```python
from build123d import *

# Parameters (mm, degrees)
F0_W     = 74
F0_H     = 32
F1_DEPTH = 3.4
F2_W     = 68.8
F2_H     = 27.8
F3_DEPTH = 10
F4_W     = 65.06
F4_H     = 24.6
F5_DEPTH = 8
F6_R     = 5
F7_R     = 1.6
F8_DEPTH = 10.001
F9_R     = 1


with BuildPart() as f1:
    # F0 (on Top) → F1 (new body)
    with BuildSketch(Plane.XY):
        Rectangle(F0_W, F0_H)
    extrude(amount=F1_DEPTH)

    # F2 (on face) → F3 (join)
    with BuildSketch(Plane.XY.offset(3.4)):
        Rectangle(F2_W, F2_H)
    extrude(amount=-F3_DEPTH)

    # F4 (on face) → F5 (cut)
    with BuildSketch(Plane.XY.offset(3.4)):
        Rectangle(F4_W, F4_H)
    extrude(amount=-F5_DEPTH, mode=Mode.SUBTRACT)

    # F6
    f6_edges = [f1.edges().sort_by_distance(p)[0] for p in [
        (-37, -16, 1.7),
        (37, -16, 1.7),
        (37, 16, 1.7),
        (-37, 16, 1.7),
    ]]
    fillet(f6_edges, radius=F6_R)

    # F7 (on face) → F8 (cut, through all)
    with BuildSketch(Plane.XY.offset(3.4)):
        with Locations((-30.004807, -10.013314)):
            Circle(F7_R)
    extrude(amount=-F8_DEPTH, mode=Mode.SUBTRACT)

    # F9
    f9_edges = [f1.edges().sort_by_distance(p)[0] for p in [
        (-34.4, 13.9, -3.3),
        (-34.4, -13.9, -3.3),
        (34.4, -13.9, -3.3),
        (34.4, 13.9, -3.3),
    ]]
    fillet(f9_edges, radius=F9_R)


solid = f1.part
```
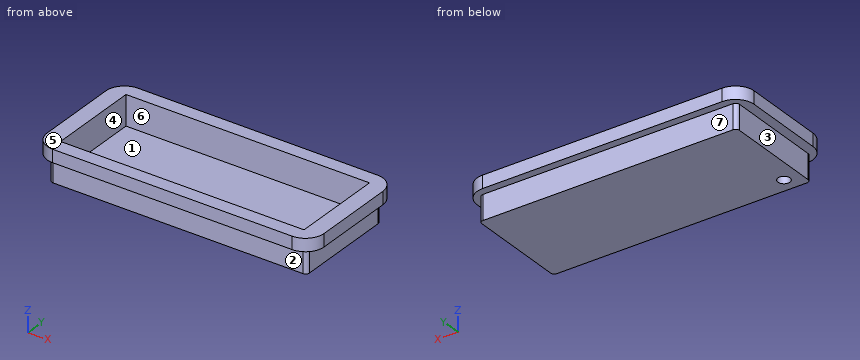
The model under review builds one solid part; all positions refer to its coordinate system, in mm. Face numbers are marked on the shaded views. A direction names the side the tool comes from. Round coordinates to 2 decimals unless told otherwise and drop trailing zeros. Write each loop counter-clockwise with the first axis right and the second up, starting at its lowest first coordinate (ties: lowest second). Pieces come first, ordered by that corner, then holes. Notation, with made-up numbers: (-26.5, 19.25) -> (15.5, 19.25) arc R13 cw to (15.5, 37.25) -> close; hole circle Ø8 at (69, 9.25). An arc over 180 degrees is marked (long way). Use CSV: the item, a comma, the result in double quotes.
Q1. To check wall thickness, follow probe 1 along X at (y, z) = (-2, -3); probe 2 along Y at (x, z) = (-14.5, -1.5); probe 3 along X at (y, z) = (0, 1.75). State the ranges of each line that lie inside material, in increasing order. Write a range as [from, to].
Checks:
probe 1,"[-34.4, -32.53], [32.53, 34.4]"
probe 2,"[-13.9, -12.3], [12.3, 13.9]"
probe 3,"[-37, -32.53], [32.53, 37]"
Q2. Consider section A-A (z = 1.75). Give the boundary of the cut face in (x, y), then the cut area to 3 significant figures.
Checks:
outline,"(-37, -11) arc R5 ccw to (-32, -16) -> (32, -16) arc R5 ccw to (37, -11) -> (37, 11) arc R5 ccw to (32, 16) -> (-32, 16) arc R5 ccw to (-37, 11) -> close; hole (-32.53, -12.3) -> (32.53, -12.3) -> (32.53, 12.3) -> (-32.53, 12.3) -> close"
area,"746 mm²"
Q3. Consider section C-C (x = 27). Give the boundary of the cut face in (y, z), then the cut area to 3 significant figures.
Checks:
outline,"(-16, 0) -> (-13.9, 0) -> (-13.9, -6.6) -> (13.9, -6.6) -> (13.9, 0) -> (16, 0) -> (16, 3.4) -> (12.3, 3.4) -> (12.3, -4.6) -> (-12.3, -4.6) -> (-12.3, 3.4) -> (-16, 3.4) -> close"
area,"95.5 mm²"
Q4. For pin 1 Ø3.5 at (x, z) = (4.5, -3.5) entering from -Y; pin 2 Ø10 at (x, y) = (18.5, -4) entering from +Z; pin 3 Ø5 at (y, z) = (12.5, -1.5) entering from +X; pin 4 Ø3 at (x, z) = (12.5, -4.5) entering from +Y, all flat-tipped, find the tip position at first contact; note any pin that passes through.
Checks:
pin 1,"y = -13.9"
pin 2,"z = -4.6"
pin 3,"x = 37"
pin 4,"y = 13.9"
Q5. Mouldability with a two-part tool opening along Y and no side actions: class the marked faces 1, 2, 3 and 4 as released by +Y, released by -Y, zero draft, split by the parting line, or undercut.
Checks:
face 1,"undercut"
face 2,"released by -Y"
face 3,"zero draft"
face 4,"undercut"
Q6. Consider section D-D (z = -2). Give the boundary of the cut face in (x, y), then the cut area to 3 significant figures.
Checks:
outline,"(-34.4, -12.9) arc R1 ccw to (-33.4, -13.9) -> (33.4, -13.9) arc R1 ccw to (34.4, -12.9) -> (34.4, 12.9) arc R1 ccw to (33.4, 13.9) -> (-33.4, 13.9) arc R1 ccw to (-34.4, 12.9) -> close; hole (-32.53, -12.3) -> (32.53, -12.3) -> (32.53, 12.3) -> (-32.53, 12.3) -> close"
area,"311 mm²"
Q7. Consider section B-B (y = 1). Give the boundary of the cut face in (x, z).
Checks:
outline,"(-37, 0) -> (-34.4, 0) -> (-34.4, -6.6) -> (34.4, -6.6) -> (34.4, 0) -> (37, 0) -> (37, 3.4) -> (32.53, 3.4) -> (32.53, -4.6) -> (-32.53, -4.6) -> (-32.53, 3.4) -> (-37, 3.4) -> close"
Q8. For the marked faces 5, 6 and 7, list the 3-axis set-ups (+Z, -Z, +X, -X, +Y, -Y) from which the entire face can be reached by the end or side of a thin tool; tool diameter is ignored.
Checks:
face 5,"+Z, +X, -X, +Y, -Y"
face 6,"+Z"
face 7,"-Z, +X, -X, +Y"
